Could you check a few things on this model? Use its own coordinates, in mm. A direction names the side the tool comes from. Give positions to 0.01 mm unless a question says otherwise; leave off trailing zeros. Order: outer loops, then holes, each group sorted by start corner. A loop starts at its lowest first (then second) coordinate and runs counter-clockwise, first axis right, second up.
from build123d import *

# Parameters (mm, degrees)
SKETCH1_W           = 10
SKETCH1_H           = 40
BOSS_EXTRUDE1_DEPTH = 1.6
CUT_EXTRUDE1_DEPTH  = 21.67752403


with BuildPart() as part:
    # Sketch1 → Boss-Extrude1 (new body)
    with BuildSketch(Plane.XY):
        Rectangle(SKETCH1_W, SKETCH1_H)
    extrude(amount=BOSS_EXTRUDE1_DEPTH)

    # Sketch3 → Cut-Extrude1 (cut, through all)
    with BuildSketch(Plane.XY.offset(1.6)):
        with BuildLine():
            Line((1.15, 12.5), (1.15, -12.5))
            ThreePointArc((1.15, -12.5), (0, -13.65), (-1.15, -12.5))
            Line((-1.15, -12.5), (-1.15, 12.5))
            ThreePointArc((-1.15, 12.5), (0, 13.65), (1.15, 12.5))
        make_face()
        with BuildLine():
            Line((1.15, 41.8), (1.15, 16.8))
            ThreePointArc((1.15, 16.8), (0, 15.65), (-1.15, 16.8))
            Line((-1.15, 16.8), (-1.15, 41.8))
            ThreePointArc((-1.15, 41.8), (0, 42.95), (1.15, 41.8))
        make_face()
        with BuildLine():
            Line((1.15, -16.8), (1.15, -41.8))
            ThreePointArc((1.15, -41.8), (0, -42.95), (-1.15, -41.8))
            Line((-1.15, -41.8), (-1.15, -16.8))
            ThreePointArc((-1.15, -16.8), (0, -15.65), (1.15, -16.8))
        make_face()
    extrude(amount=-CUT_EXTRUDE1_DEPTH, mode=Mode.SUBTRACT)


solid = part.part
Item 1: Imagine slicing it at C-C on y = 5. List the corners of the cut face in (x, z) for me.
Findings:
outline: (-5, 0) - (-1.15, 0) - (-1.15, 1.6) - (-5, 1.6) - close; (1.15, 0) - (5, 0) - (5, 1.6) - (1.15, 1.6) - close
Item 2: For faces 1 (the flat face through (-2, 0, 1.6)), 2 (the flat face through (-1.15, 18, 1)), 3 (the flat face through (1.15, 0, 1)), 4 (the flat face through (-1.15, -18, 1)), 5 (the flat face through (-3, -20, 1)), which set-ups out of +Z, -Z, +X, -X, +Y, -Y let a thin tool reach every point of the face, with its end or its side?
Findings:
face 1: +Z, +X, -X, +Y, -Y
face 2: +Z, -Z, +Y
face 3: +Z, -Z
face 4: +Z, -Z, -Y
face 5: +Z, -Z, +X, -X, -Y
Item 3: We'd pull the mould along X, two halves only. Please class faces 6 (the flat face through (-5, 0, 1)), 7 (the flat face through (5, 0, 1)), 8 (the flat face through (1.15, 18, 1)), 9 (the flat face through (3, -20, 1)): +X half, -X half, draft (parallel to the pull), parting line (faces both ways), or undercut.
Findings:
face 6: -X half
face 7: +X half
face 8: undercut
face 9: draft
Item 4: Please list where these lines run through material, in increasing order: line 1 along X through (y, z) = (-6.5, 0.15); line 2 along X through (y, z) = (-13.5, 0.9); line 3 along Y through (x, z) = (1, 1.4).
Findings:
line 1: x = -5 to -1.15, 1.15 to 5
line 2: x = -5 to -0.57, 0.57 to 5
line 3: y = -16.23 to -13.07, 13.07 to 16.23
Item 5: Imagine slicing it at B-B on z = 0.45. List the corners of the cut face in (x, y) for me, then the cut area to 3 significant figures.
Findings:
outline: (-5, -20) - (-1.15, -20) - (-1.15, -16.8) arc R1.15 cw to (1.15, -16.8) - (1.15, -20) - (5, -20) - (5, 20) - (1.15, 20) - (1.15, 16.8) arc R1.15 cw to (-1.15, 16.8) - (-1.15, 20) - (-5, 20) - close; hole (-1.15, -12.5) arc R1.15 ccw to (1.15, -12.5) - (1.15, 12.5) arc R1.15 ccw to (-1.15, 12.5) - close
area: 319 mm2
Item 6: Imagine slicing it at A-A on x = 0. List the corners of the cut face in (y, z) for me, then the cut area to 3 significant figures.
Findings:
outline: (-15.65, 0) - (-13.65, 0) - (-13.65, 1.6) - (-15.65, 1.6) - close; (13.65, 0) - (15.65, 0) - (15.65, 1.6) - (13.65, 1.6) - close
area: 6.40 mm2
